The listing builds one solid part. Answer for the finished solid, in the listing's coordinates (mm). A direction names the side the tool comes from. Give positions to 0.01 mm unless a question says otherwise; leave off trailing zeros. Write each loop counter-clockwise with the first axis right and the second up, starting at its lowest first coordinate (ties: lowest second). Pieces come first, ordered by that corner, then holes. Notation, with made-up numbers: (88.25, 0.5) - (102.25, 0.5) arc R26 ccw to (102.25, 26.5) - close; hole circle Ø2 at (-33, 75). An arc over 180 degrees is marked (long way). Answer in a Markdown table with one row per item. Add a question column.
from build123d import *

# Parameters (mm, degrees)
F0_R     = 11.1
F1_DEPTH = 1.75
F2_DEPTH = 5


with BuildPart() as f1:
    # F0 (on Top) → F1 (new body, symmetric)
    with BuildSketch(Plane.XY):
        with BuildLine():
            Line((6, 38.218746), (0, 38.218746))
            Line((0, 38.218746), (-6, 38.218746))
            Line((-6, 38.218746), (-10.109618, 16.405044))
            ThreePointArc((-10.109618, 16.405044), (-13.665242, 7.889631), (-19.261994, 0.552664))
            Line((-19.261994, 0.552664), (-36.098405, -13.91322))
            Line((-36.098405, -13.91322), (-33.098405, -19.109373))
            Line((-33.098405, -19.109373), (-30.098405, -24.305525))
            Line((-30.098405, -24.305525), (-9.152376, -16.957708))
            ThreePointArc((-9.152376, -16.957708), (0, -15.779262), (9.152376, -16.957708))
            Line((9.152376, -16.957708), (30.098405, -24.305525))
            Line((30.098405, -24.305525), (33.098405, -19.109373))
            Line((33.098405, -19.109373), (36.098405, -13.91322))
            Line((36.098405, -13.91322), (19.261994, 0.552664))
            ThreePointArc((19.261994, 0.552664), (13.665242, 7.889631), (10.109618, 16.405044))
            Line((10.109618, 16.405044), (6, 38.218746))
        make_face()
        Polygon((-30.500328, -17.609373), (-32.256535, -14.567534), (-20.051088, -4.080584), (-13.559434, -15.32446), (-28.744122, -20.651212), align=None, mode=Mode.SUBTRACT)
        with BuildLine():
            Line((-9.885613, -14.565564), (-11.332004, -15.072955))
            Line((-11.332004, -15.072955), (-18.719564, -2.277326))
            Line((-18.719564, -2.277326), (-17.556955, -1.27841))
            ThreePointArc((-17.556955, -1.27841), (-16.789561, -0.483972), (-16.045193, 0.33208))
            Line((-16.045193, 0.33208), (-7.735007, -14.061585))
            ThreePointArc((-7.735007, -14.061585), (-8.813913, -14.2982), (-9.885613, -14.565564))
        make_face(mode=Mode.SUBTRACT)
        Circle(F0_R, mode=Mode.SUBTRACT)
        Polygon((30.500328, -17.609373), (28.744122, -20.651212), (13.559434, -15.32446), (20.051088, -4.080584), (32.256535, -14.567534), align=None, mode=Mode.SUBTRACT)
        with BuildLine():
            Line((17.556955, -1.27841), (18.719564, -2.277326))
            Line((18.719564, -2.277326), (11.332004, -15.072955))
            Line((11.332004, -15.072955), (9.885613, -14.565564))
            ThreePointArc((9.885613, -14.565564), (8.813913, -14.2982), (7.735007, -14.061585))
            Line((7.735007, -14.061585), (16.045193, 0.33208))
            ThreePointArc((16.045193, 0.33208), (16.789561, -0.483972), (17.556955, -1.27841))
        make_face(mode=Mode.SUBTRACT)
        with BuildLine():
            Line((8.310186, 13.729505), (-8.310186, 13.729505))
            ThreePointArc((-8.310186, 13.729505), (-7.975648, 14.782172), (-7.671342, 15.843974))
            Line((-7.671342, 15.843974), (-7.38756, 17.350281))
            Line((-7.38756, 17.350281), (7.38756, 17.350281))
            Line((7.38756, 17.350281), (7.671342, 15.843974))
            ThreePointArc((7.671342, 15.843974), (7.975648, 14.782172), (8.310186, 13.729505))
        make_face(mode=Mode.SUBTRACT)
        Polygon((6.491654, 19.405044), (-6.491654, 19.405044), (-3.512413, 35.218746), (0, 35.218746), (3.512413, 35.218746), align=None, mode=Mode.SUBTRACT)
    extrude(amount=F1_DEPTH, both=True)

    # F0 (on Top) → F2 (join, symmetric)
    with BuildSketch(Plane.XY):
        Polygon((13.559434, -15.32446), (28.744122, -20.651212), (30.500328, -17.609373), (32.256535, -14.567534), (20.051088, -4.080584), align=None)
        Polygon((-3.512413, 35.218746), (-6.491654, 19.405044), (6.491654, 19.405044), (3.512413, 35.218746), (0, 35.218746), align=None)
        Polygon((-20.051088, -4.080584), (-32.256535, -14.567534), (-30.500328, -17.609373), (-28.744122, -20.651212), (-13.559434, -15.32446), align=None)
    extrude(amount=F2_DEPTH, both=True)


solid = f1.part
1. Section C-C (z = -0.25) is taken. State how many separate pieces and enclosed holes the cut face has, and give its area (3 significant figures).
2. Straight lines are drawn through the part: L1, parallel to X at y = -2, z = 0.25; L2, parallel to X at y = -7.5, z = -0.25; L3, parallel to X at y = 14.5, z = -1. For each, find the intervals that lie inside material, in ascending order. Write a range as [from, to].
3. A tool of negligible diameter and unlimited length cuts with its end or side. For faces 1 (the face through (-14.974, -8.765, 0.024)), 2 (the face through (-21.258, -18.025, -3.352)), 3 (the face through (-26.07, -9.25, -3.35)), from which of +Z, -Z, +X, -X, +Y, -Y can it reach the whole face along a straight path? Write none if from no direction.
4. Section D-D (y = 6) is taken. Give the vertices of the cut face in (x, z), and give its area (3 significant figures).
5. Given pin 1 Ø2.5 at (x, z) = (1, 4) entering from -Y; pin 2 Ø1 at (x, z) = (0.5, 3) entering from +Y; pin 3 Ø1 at (x, z) = (-3.5, -0.5) entering from -Y, each flat-ended and moving along its own axis, determine where each tip first touches the part or whether it passes through.
6. Section A-A (z = -4) is taken. Give the vertices of the cut face in (x, y).
7. Section B-B (x = 0) is taken. Give the vertices of the cut face in (y, z).
Geometry check:
| question | item | result |
|---|---|---|
| 1 | separate pieces | 1 |
| 1 | enclosed holes | 4 |
| 1 | area | 1,420 mm² |
| 2 | L1 | [-22.23, -18.4], [-14.7, -10.92], [10.92, 14.7], [18.4, 22.23] |
| 2 | L2 | [-28.63, -15.7], [-11.52, -8.18], [8.18, 11.52], [15.7, 28.63] |
| 2 | L3 | [-10.69, -8.06], [8.06, 10.69] |
| 3 | face 1 | +Z, -Z |
| 3 | face 2 | -Z, -Y |
| 3 | face 3 | -Z, -X, +Y |
| 4 | outline | (-14.84, -1.75) - (-9.34, -1.75) - (-9.34, 1.75) - (-14.84, 1.75) - close; (9.34, -1.75) - (14.84, -1.75) - (14.84, 1.75) - (9.34, 1.75) - close |
| 4 | area | 38.5 mm² |
| 5 | pin 1 | y = 19.41 |
| 5 | pin 2 | y = 35.22 |
| 5 | pin 3 | y = -16 |
| 6 | outline | (-32.26, -14.57) - (-30.5, -17.61) - (-28.74, -20.65) - (-13.56, -15.32) - (-20.05, -4.08) - close; (-6.49, 19.41) - (6.49, 19.41) - (3.51, 35.22) - (-3.51, 35.22) - close; (13.56, -15.32) - (28.74, -20.65) - (30.5, -17.61) - (32.26, -14.57) - (20.05, -4.08) - close |
| 7 | outline | (-15.78, -1.75) - (-11.1, -1.75) - (-11.1, 1.75) - (-15.78, 1.75) - close; (11.1, -1.75) - (13.73, -1.75) - (13.73, 1.75) - (11.1, 1.75) - close; (17.35, -1.75) - (19.41, -1.75) - (19.41, -5) - (35.22, -5) - (35.22, -1.75) - (38.22, -1.75) - (38.22, 1.75) - (35.22, 1.75) - (35.22, 5) - (19.41, 5) - (19.41, 1.75) - (17.35, 1.75) - close |
